Geometry check sheet. Reference: the model listing, model coordinates, mm. A direction names the side the tool comes from. Round coordinates to 2 decimals unless told otherwise and drop trailing zeros. Write each loop counter-clockwise with the first axis right and the second up, starting at its lowest first coordinate (ties: lowest second). Pieces come first, ordered by that corner, then holes.
Item 1: Cross-section at B-B (y = -31). Enter the section's corners in (x, z), then the cut area to 3 significant figures.
Item 2: Access from +Z, -Z, +X, -X, +Y, -Y to the whole of each face (thin tool, end or side, straight path). Record for faces 1 (the face through (-40, 5, 5)), 2 (the face through (40, -5, 5)), 3 (the face through (45, 0, 5)).
Item 3: Scan line: probe 1 along Y at (x, z) = (40, 8). Record every from-to range of solid material in increasing order.
Item 4: Depth check by flat-ended pin: P1, Ø3, axis at y = -8.5, z = 6.5, coming from the +X side; P2, Ø3, axis at y = -28.5, z = 3, coming from the -X side. Enter the tip coordinate at first touch or a pass-through.
Item 5: Cross-section at A-A (z = 5). Enter the section's corners in (x, y).
Item 6: Draft check along Y on faces 4 (the face through (45, -40, 5)), 5 (the face through (35, -30, 5)), 6 (the face through (-1, -45, 5)). Enter one of: pulls with the +Y half, pulls with the -Y half, needs draft (parallel to the pull), parting line crosses it, or undercut.
from build123d import *

# Parameters (mm, degrees)
F1_DEPTH = 10


with BuildPart() as f1:
    # F0 (on Top) → F1 (new body)
    with BuildSketch(Plane.XY):
        Polygon((0, -45), (45, -45), (45, -35), (35, -35), (35, -25), (45, -25), (45, -15), (35, -15), (35, -5), (45, -5), (45, 5), (35, 5), (35, 15), (45, 15), (45, 25), (35, 25), (-35, 25), (-45, 25), (-45, 15), (-35, 15), (-35, 5), (-45, 5), (-45, -5), (-35, -5), (-35, -15), (-45, -15), (-45, -25), (-35, -25), (-35, -35), (-45, -35), (-45, -45), align=None)
    extrude(amount=F1_DEPTH)


solid = f1.part
Resolved:
1. outline: (-35, 0) - (35, 0) - (35, 10) - (-35, 10) - close
1. area: 700 mm2
2. face 1: +Z, -Z, -X
2. face 2: +Z, -Z, +X
2. face 3: +Z, -Z, +X, +Y, -Y
3. probe 1: y = -45 to -35, -25 to -15, -5 to 5, 15 to 25
4. P1: stops at x = 35
4. P2: stops at x = -35
5. outline: (-45, -45) - (45, -45) - (45, -35) - (35, -35) - (35, -25) - (45, -25) - (45, -15) - (35, -15) - (35, -5) - (45, -5) - (45, 5) - (35, 5) - (35, 15) - (45, 15) - (45, 25) - (-45, 25) - (-45, 15) - (-35, 15) - (-35, 5) - (-45, 5) - (-45, -5) - (-35, -5) - (-35, -15) - (-45, -15) - (-45, -25) - (-35, -25) - (-35, -35) - (-45, -35) - close
6. face 4: needs draft
6. face 5: undercut
6. face 6: pulls with the -Y half
